The listing builds one solid part. Answer for the finished solid, in the listing's coordinates (mm). Face numbers are marked on the shaded views. Round coordinates to 2 decimals unless told otherwise and drop trailing zeros. Order: outer loops, then holes, each group sorted by start corner. A loop starts at its lowest first (then second) coordinate and runs counter-clockwise, first axis right, second up. Notation, with made-up numbers: (35, -9) - (71, -9) arc R23 ccw to (71, 17) - close; hole circle Ø2 at (-12, -11). An arc over 180 degrees is marked (long way). One line per item, written item: value. Start each with the question number.
1. Straight lines are drawn through the part: line 1 (Y direction, x = 10.75, z = 42.5) (3 decimals); line 2 (Z direction, x = 5.5, y = 70); line 3 (Y direction, x = 16, z = -4) (3 decimals). For each, find the intervals that lie inside material, in ascending order.
2. Section A-A, the plane z = 41 is taken. Give the vertices of the cut face in (x, y) (3 decimals).
3. Section B-B, the plane x = 5.5 is taken. Give the vertices of the cut face in (y, z) (3 decimals), then the cut area to 3 significant figures.
4. Section C-C, the plane y = 59 is taken. Give the vertices of the cut face in (x, z), then the cut area to 3 significant figures.
5. For a pull along Z with two mould halves and no side action, classify the marked faces 1, 2, 3 and 4 as released by +Z, released by -Z, zero draft, split by the parting line, or undercut.
6. Flat-ended cylindrical pins translate along their axes: P1, Ø8, axis at x = 17.5, y = 47, coming from the -Z side; P2, Ø3, axis at x = 6.5, z = 14, coming from the +Y side; P3, Ø2, axis at x = 13.5, y = 78, coming from the -Z side. Find the tip coordinate at first contact, or state that the pin passes through.
7. Section D-D, the plane z = 11 is taken. Give the vertices of the cut face in (x, y) (3 decimals), then the cut area to 3 significant figures.
from build123d import *

# Parameters (mm, degrees)
F1_DEPTH = 25.4
F2_R     = 1.27
F3_R     = 1.27


with BuildPart() as f1:
    # F0 (on Right) → F1 (new body)
    with BuildSketch(Plane.YZ):
        Polygon((0, -35.935552), (0, 49.789448), (77.47, 49.789448), (77.47, 39.629448), (77.47, 34.549448), (80.645, 34.549448), (80.645, 49.789448), (80.645, 52.964448), (77.47, 52.964448), (0, 52.964448), (-3.175, 52.964448), (-3.175, 49.789448), (-3.175, 11.689448), (-3.175, -35.935552), align=None)
        Polygon((77.47, 34.549448), (77.47, 39.629448), (74.93, 39.629448), align=None)
    extrude(amount=F1_DEPTH)

    # F2
    f2_edges = [f1.edges().sort_by_distance(p)[0] for p in [
        (25.4, 38.735, 52.964448),
        (0, 38.735, 52.964448),
        (12.7, 80.645, 52.964448),
        (25.4, 80.645, 43.756948),
        (12.7, 80.645, 34.549448),
        (0, 80.645, 43.756948),
        (25.4, -1.5875, -35.935552),
        (0, -1.5875, -35.935552),
    ]]
    fillet(f2_edges, radius=F2_R)

    # F3
    f3_edges = [f1.edges().sort_by_distance(p)[0] for p in [
        (12.7, 0, 49.789448),
        (12.7, 77.47, 49.789448),
    ]]
    fillet(f3_edges, radius=F3_R)


solid = f1.part
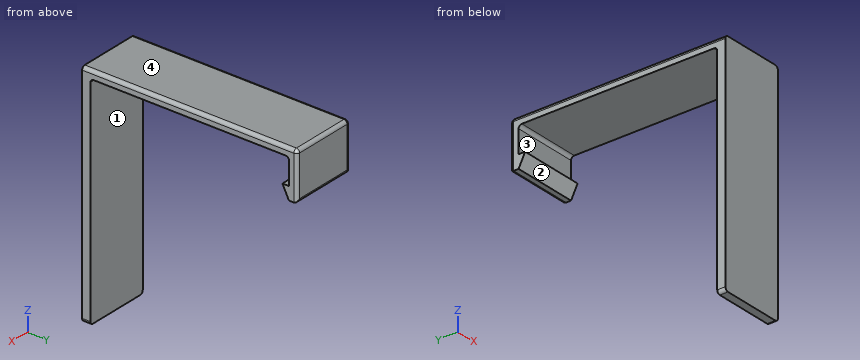
Answer list:
1. line 1: y = -3.175 to 0, 77.47 to 80.645
1. line 2: z = 49.79 to 52.96
1. line 3: y = -3.175 to 0
2. outline: (0, -3.175) - (25.4, -3.175) - (25.4, 0) - (0, 0) - close; (0, 77.47) - (25.4, 77.47) - (25.4, 79.375) arc R1.27 ccw to (24.13, 80.645) - (1.27, 80.645) arc R1.27 ccw to (0, 79.375) - close
3. outline: (-3.175, -35.936) - (0, -35.936) - (0, 48.519) arc R1.27 cw to (1.27, 49.789) - (76.2, 49.789) arc R1.27 cw to (77.47, 48.519) - (77.47, 39.629) - (74.93, 39.629) - (77.47, 34.549) - (79.375, 34.549) arc R1.27 ccw to (80.645, 35.819) - (80.645, 51.694) arc R1.27 ccw to (79.375, 52.964) - (-3.175, 52.964) - close
3. area: 593 mm²
4. outline: (0, 49.79) - (25.4, 49.79) - (25.4, 51.69) arc R1.27 ccw to (24.13, 52.96) - (1.27, 52.96) arc R1.27 ccw to (0, 51.69) - close
4. area: 80.0 mm²
5. face 1: zero draft
5. face 2: released by -Z
5. face 3: undercut
5. face 4: released by +Z
6. P1: stops at z = 49.79
6. P2: stops at y = 0
6. P3: stops at z = 34.55
7. outline: (0, -3.175) - (25.4, -3.175) - (25.4, 0) - (0, 0) - close
7. area: 80.6 mm²
